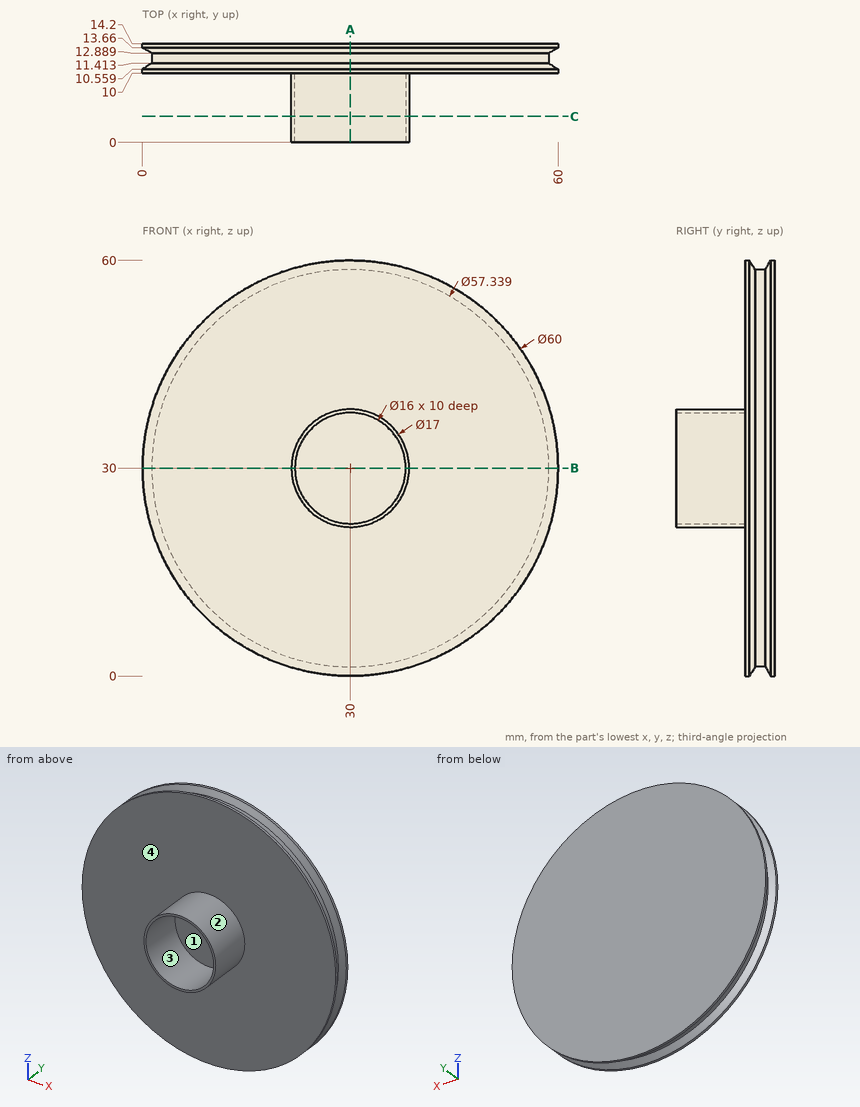
For this review, use the dimensioned drawing (mm, ordinates from the lowest corner) and the shaded views. Round coordinates to 2 decimals unless told otherwise and drop trailing zeros. Order: outer loops, then holes, each group sorted by start corner. A loop starts at its lowest first (then second) coordinate and runs counter-clockwise, first axis right, second up. Notation, with made-up numbers: (69, 57) - (73, 57) arc R27 ccw to (73, 93) - close; hole circle Ø2 at (-39.5, -8.75). An arc over 180 degrees is marked (long way). Use one line per item in the form item = value.
Q1. Mouldability with a two-part tool opening along X and no side actions: class the marked faces 1, 2, 3 and 4 as pulls with the +X half, pulls with the -X half, needs draft (parallel to the pull), parting line crosses it, or undercut.
Response values:
face_1 = undercut
face_2 = parting line crosses it
face_3 = undercut
face_4 = needs draft
Q2. Add section B-B on z = 30. Give the boundary of the cut face in (x, y).
Response values:
outline = (0, 10) - (21.5, 10) - (21.5, 0) - (22, 0) - (22, 10) - (38, 10) - (38, 0) - (38.5, 0) - (38.5, 10) - (60, 10) - (60, 10.56) - (58.67, 11.41) - (58.67, 12.89) - (60, 13.66) - (60, 14.2) - (0, 14.2) - (0, 13.66) - (1.33, 12.89) - (1.33, 11.41) - (0, 10.56) - close
Q3. Add section C-C on y = 3.75. Give the boundary of the cut face in (x, z).
Response values:
outline = circle Ø17 at (30, 30); hole circle Ø16 at (30, 30)
Q4. Add section A-A on x = 30. Give the boundary of the cut face in (y, z), then the cut area to 3 significant figures.
Response values:
outline = (0, 21.5) - (10, 21.5) - (10, 0) - (10.56, 0) - (11.41, 1.33) - (12.89, 1.33) - (13.66, 0) - (14.2, 0) - (14.2, 60) - (13.66, 60) - (12.89, 58.67) - (11.41, 58.67) - (10.56, 60) - (10, 60) - (10, 38.5) - (0, 38.5) - (0, 38) - (10, 38) - (10, 22) - (0, 22) - close
area = 256 mm^2
Q5. To check wall thickness, follow line 1 (Z direction, x = 30, y = 2); line 2 (Y direction, x = 16, z = 6); line 3 (X direction, y = 2, z = 26). State the ranges of each line that lie inside material, in increasing order.
Response values:
line_1 = 21.5 to 22, 38 to 38.5
line_2 = 10 to 14.2
line_3 = 22.5 to 23.07, 36.93 to 37.5
Q6. Clearance check with flat-ended pins moving along their axes: P1, Ø1, axis at x = 26, z = 44, coming from the -Y side; P2, Ø2, axis at x = 33.5, y = 8, coming from the +Z side; P3, Ø6, axis at y = 5.5, z = 24, coming from the +X side. State where each tip first meets the part, or that it passes through.
Response values:
P1 = 10
P2 = 38.12
P3 = 37.95
